```python
from build123d import *

# Parameters (mm, degrees)
F1_DEPTH = 1.6


# Not quite as in the source:
# - a feature names something its author has since deleted; it is built from what else it names


with BuildPart() as f1:
    # F0 (on Right) → F1 (new body, symmetric)
    with BuildSketch(Plane.YZ):
        with BuildLine():
            Line((-27.5, 0), (-27.5, -3.2))
            Line((-27.5, -3.2), (-24.3, -3.2))
            Line((-24.3, -3.2), (-24.3, 0))
            add(Edge.make_bspline(
                [(-24.3, 0), (-15.858107704, 2.1141811864), (-0.2087572903, 6.0333927878), (11.9158815387, 1.9025152075), (17.5, 0)],
                knots=[0, 0, 0, 0, 0.5394404287, 1, 1, 1, 1], degree=3))
            Line((17.5, 0), (17.5, -3.2))
            Line((17.5, -3.2), (27.5, -3.2))
            Line((27.5, -3.2), (27.5, 0))
            Line((27.5, 0), (27.5, 10.5))
            Line((27.5, 10.5), (17.5, 10.5))
            Line((17.5, 10.5), (17.5, 13.7))
            Line((17.5, 13.7), (27.5, 13.7))
            Line((27.5, 13.7), (27.5, 55.6200032))
            Line((27.5, 55.6200032), (39, 68.5000032))
            Line((39, 68.5000032), (39, 71.7))
            Line((39, 71.7), (-11, 15.7))
            Line((-11, 15.7), (-11, 18.7))
            Line((-11, 18.7), (-17.5, 13.7))
            Line((-17.5, 13.7), (-17.5, 10.5))
            Line((-17.5, 10.5), (-27.5, 10.5))
            Line((-27.5, 10.5), (-27.5, 0))
        make_face()
    extrude(amount=F1_DEPTH, both=True)


solid = f1.part
```
Part model, mm, in its own coordinate system. A direction names the side the tool comes from. Round coordinates to 2 decimals unless told otherwise and drop trailing zeros. Write each loop counter-clockwise with the first axis right and the second up, starting at its lowest first coordinate (ties: lowest second). Pieces come first, ordered by that corner, then holes.
Item 1: Cut at A-A, the plane y = 21. Give the cut face in (x, z).
Results:
outline: (-1.6, -3.2) - (1.6, -3.2) - (1.6, 10.5) - (-1.6, 10.5) - close; (-1.6, 13.7) - (1.6, 13.7) - (1.6, 51.54) - (-1.6, 51.54) - close
Item 2: Cut at B-B, the plane z = 17.5. Give the cut face in (x, y), plus the area to 3 significant figures.
Results:
outline: (-1.6, -12.56) - (1.6, -12.56) - (1.6, -11) - (-1.6, -11) - close; (-1.6, -9.39) - (1.6, -9.39) - (1.6, 27.5) - (-1.6, 27.5) - close
area: 123 mm2
Item 3: Cut at C-C, the plane y = 33. Give the cut face in (x, z), plus the area to 3 significant figures.
Results:
outline: (-1.6, 61.78) - (1.6, 61.78) - (1.6, 64.98) - (-1.6, 64.98) - close
area: 10.2 mm2
Item 4: Which spindle directions (+Z, -Z, +X, -X, +Y, -Y) get a long thin tool onto all of the face, cutting with end or side? Do faces 4 (the flat face through (1.6, 8, 18)), 5 (the flat face through (0, -24.3, -2)), 6 (the flat face through (0, -17.5, 12)), 7 (the flat face through (0, 22, 13.7)), 8 (the flat face through (0, 27.5, 4)). Say none if no direction does.
Results:
face 4: +Z, -Z, +X, +Y, -Y
face 5: -Z, +X, -X
face 6: +Z, +X, -X, -Y
face 7: +X, -X, +Y
face 8: -Z, +X, -X, +Y
Item 5: Two-plate mould, pull along Y, no slides. Class faces 1 (the flat face through (0, 17.5, 12)), 2 (the flat face through (0, -11, 17)), 3 (the flat face through (0, -26, -3.2)): +Y half, -Y half, draft (parallel to the pull), parting line (faces both ways), or undercut.
Results:
face 1: +Y half
face 2: undercut
face 3: draft
Item 6: Cut at D-D, the plane z = 46. Give the cut face in (x, y), plus the area to 3 significant figures.
Results:
outline: (-1.6, 16.05) - (1.6, 16.05) - (1.6, 27.5) - (-1.6, 27.5) - close
area: 36.6 mm2
Item 7: Probe L1, parallel to Y at x = 0.2, z = 32.5; L2, parallel to Y at x = -0.85, z = 9.5; L3, parallel to Z at x = 0.7, y = 25.5. List the from-to ranges inside material, lowest first.
Results:
L1: y = 4 to 27.5
L2: y = -27.5 to 27.5
L3: z = -3.2 to 10.5, 13.7 to 56.58
Item 8: Drop flat-ended pins along their axis: pin 1 Ø1.5 at (x, z) = (-0.5, 17) entering from +Y; pin 2 Ø1.6 at (x, y) = (0.5, -20.5) entering from +Z; pin 3 Ø3 at (y, z) = (-10, 20) entering from +X; pin 4 Ø1.6 at (x, y) = (0, 21) entering from +Z. Give the stop position or say it passes through.
Results:
pin 1: stops at y = 27.5
pin 2: stops at z = 10.5
pin 3: passes through
pin 4: stops at z = 52.44
